from build123d import *

# Parameters (mm, degrees)
SKETCH1_R           = 1.016
BOSS_EXTRUDE1_DEPTH = 1.27
SKETCH2_R           = 1.016
BOSS_EXTRUDE3_DEPTH = 63.5


with BuildPart() as part:
    # Sketch1 → Boss-Extrude1 (new body)
    with BuildSketch(Plane.XY):
        Polygon((-36.869116619, 17.792333901), (-36.869116619, -0.749666099), (-5.119116619, -0.749666099), (-5.119116619, 6.870333901), (-31.789116619, 6.870333901), (-31.789116619, 17.792333901), align=None)
        with Locations((-34.329116619, 13.982333901)):
            Circle(SKETCH1_R, mode=Mode.SUBTRACT)
        with Locations((-34.329116619, 3.060333901)):
            Circle(SKETCH1_R, mode=Mode.SUBTRACT)
        with Locations((-7.659116619, 3.060333901)):
            Circle(SKETCH1_R, mode=Mode.SUBTRACT)
    extrude(amount=BOSS_EXTRUDE1_DEPTH)

    # Sketch2 → Boss-Extrude3 (add)
    with BuildSketch(Plane.XY.offset(1.27)):
        with BuildLine():
            Line((-34.329116619, 5.600333901), (-7.659116619, 5.600333901))
            ThreePointArc((-7.659116619, 5.600333901), (-5.119116619, 3.060333901), (-7.659116619, 0.520333901))
            Line((-7.659116619, 0.520333901), (-34.329116619, 0.520333901))
            ThreePointArc((-34.329116619, 0.520333901), (-36.869116619, 3.060333901), (-34.329116619, 5.600333901))
        make_face()
        with Locations((-34.329116619, 3.060333901)):
            Circle(SKETCH2_R, mode=Mode.SUBTRACT)
        with Locations((-7.659116619, 3.060333901)):
            Circle(SKETCH2_R, mode=Mode.SUBTRACT)
    extrude(amount=BOSS_EXTRUDE3_DEPTH)


solid = part.part
Input: part model. Units: mm. Frame: model coordinates. A direction names the side the tool comes from. Coordinates: 2 decimals unless noted, no trailing zeros. Loops run counter-clockwise (first coordinate to the right, second up) from the corner with the lowest first, then second, coordinate; pieces in that order, holes last. Notation, with made-up numbers: (43.5, 60.25) -> (63.5, 60.25) arc R21 cw to (63.5, 73.25) -> close; hole circle Ø1 at (-22, -8.5). An arc over 180 degrees is marked (long way). Write each question's results on one line, items separated by ' | '. Start each with the question number.
Q1. Ray query, line 1 (Y direction, x = -30.5, z = 45); line 2 (X direction, y = 3.25, z = 6); line 3 (Z direction, x = -17.5, y = 6.5). Return the intervals inside material, ascending. Write a range as from..to.
Q2. Reachability of faces 4 (the flat face through (-21, 0.52, 33)), 5 (the cylindrical face through (-5.12, 3.12, 32.58)), 6 (the flat face through (-21, 5.6, 33)), 7 (the cylindrical face through (-36.87, 3, 32.58)) from +Z, -Z, +X, -X, +Y, -Y: full face, straight path, thin tool, end or side. Return the list, or none.
Q3. Pin query (flat end, axial travel): pin 1 (13.5 mm diameter, centred on x = -20.5, z = 23, fed in from +Y); pin 2 (5 mm diameter, centred on x = -27, y = 7, fed in from -Z); pin 3 (0.6 mm diameter, centred on x = -18, z = 1, fed in from +Y); pin 4 (3 mm diameter, centred on x = -19.5, z = 27.5, fed in from -Y). Return the tip coordinate at first contact, or that it passes through.
Q4. Section B-B, the plane x = -12. Return the cut outline in (y, z).
Q5. Section C-C, the plane y = 11.5. Return the cut outline in (x, z).
Q6. Pull-direction query (Y, two-part tool) for faces 1 (the cylindrical face through (-8.408, 3.747, 31.932)), 2 (the flat face through (-24.7, 6.6, 0)), 3 (the flat face through (-34, 17.792, 1)); classes: released by +Y, released by -Y, zero draft, split by the parting line, or undercut.
Q7. Section A-A, the plane z = 58. Return the cut outline in (x, y).
Found:
1) line 1: 0.52..5.6 | line 2: -36.86..-35.33, -33.33..-8.66, -6.66..-5.13 | line 3: 0..1.27
2) face 4: +Z, +X, -X, -Y | face 5: +Z, +X | face 6: +Z, +X, -X, +Y | face 7: +Z, -X
3) pin 1: y = 5.6 | pin 2: z = 0 | pin 3: y = 6.87 | pin 4: y = 0.52
4) outline: (-0.75, 0) -> (6.87, 0) -> (6.87, 1.27) -> (5.6, 1.27) -> (5.6, 64.77) -> (0.52, 64.77) -> (0.52, 1.27) -> (-0.75, 1.27) -> close
5) outline: (-36.87, 0) -> (-31.79, 0) -> (-31.79, 1.27) -> (-36.87, 1.27) -> close
6) face 1: undercut | face 2: zero draft | face 3: released by +Y
7) outline: (-34.33, 0.52) -> (-7.66, 0.52) arc R2.54 ccw to (-7.66, 5.6) -> (-34.33, 5.6) arc R2.54 ccw to start; hole circle Ø2.03 at (-34.33, 3.06); hole circle Ø2.03 at (-7.66, 3.06)
